```python
from build123d import *

# Parameters (mm, degrees)
F0_R     = 1.8
F0_R_2   = 1.3
F1_DEPTH = 13
F0_W     = 30
F0_H     = 12
F2_DEPTH = 3
F0_W_2   = 90
F0_H_2   = 90
F3_DEPTH = 2


with BuildPart() as f1:
    # F0 (on Top) → F1 (new body)
    with BuildSketch(Plane.XY):
        with Locations((-35, 0)):
            Circle(F0_R)
        with Locations((-35, 0)):
            Circle(F0_R_2, mode=Mode.SUBTRACT)
    extrude(amount=F1_DEPTH)



with BuildPart() as f1b:
    # F0 (on Top) → F1, piece 2 (new body)
    with BuildSketch(Plane.XY):
        with Locations((-20, 0)):
            Circle(F0_R)
        with Locations((-20, 0)):
            Circle(F0_R_2, mode=Mode.SUBTRACT)
    extrude(amount=F1_DEPTH)


with BuildPart() as f1_1:
    add(f1.part)

    add(f1b.part)  # F2 merges F1b
    # F0 (on Top) → F2 (join)
    with BuildSketch(Plane.XY):
        with Locations((-27, 0)):
            Rectangle(F0_W, F0_H)
        with Locations((-35, 0)):
            Circle(F0_R, mode=Mode.SUBTRACT)
        with Locations((-20, 0)):
            Circle(F0_R, mode=Mode.SUBTRACT)
        with Locations((-20, 0)):
            Circle(F0_R_2)
        with Locations((-35, 0)):
            Circle(F0_R_2)
    extrude(amount=F2_DEPTH)

    # F0 (on Top) → F3 (join)
    with BuildSketch(Plane.XY):
        Rectangle(F0_W_2, F0_H_2)
        with Locations((-27, 0)):
            Rectangle(F0_W, F0_H, mode=Mode.SUBTRACT)
    extrude(amount=F3_DEPTH)


solid = f1_1.part
```
For this review, take the finished solid that the model builds, in its own axes (mm). A direction names the side the tool comes from. Coordinates: 2 decimals unless noted, no trailing zeros. Loops run counter-clockwise (first coordinate to the right, second up) from the corner with the lowest first, then second, coordinate; pieces in that order, holes last.
1. Add section B-B, the plane x = -20. Give the boundary of the cut face in (y, z).
2. Insertion check: P1, Ø1.1, axis at x = -21, z = 2.5, coming from the -Y side; P2, Ø1.3, axis at x = -34.5, y = 0, coming from the +Z side; P3, Ø0.5, axis at y = -1, z = 2.5, coming from the -X side; P4, Ø6, axis at x = 0, y = -34.5, coming from the +Z side. Each pin has a flat end and moves straight along its axis. Give the tip position at first contact, or say it passes through.
3. Mouldability with a two-part tool opening along X and no side actions: class faces 3 (the flat face through (-1, 45, 1)), 4 (the flat face through (-35, 0, 3)), 5 (the flat face through (45, -1, 1)) as +X half, -X half, draft (parallel to the pull), parting line (faces both ways), or undercut.
4. Add section C-C, the plane y = 0. Give the boundary of the cut face in (x, z), then the cut area to 3 significant figures.
5. For faces 1 (the flat face through (-1, 1, 0)), 2 (the cylindrical face through (-33.283, 0.541, 7.93)), list the 3-axis set-ups (+Z, -Z, +X, -X, +Y, -Y) from which the entire face can be reached by the end or side of a thin tool; tool diameter is ignored.
6. For line 1 (Y direction, x = -35, z = 9); line 2 (Z direction, x = -41, y = -28.5); line 3 (Z direction, x = -22, y = 2), list the stretches that pass through material, from the lowest coordinate up.
7. Add section D-D, the plane x = -5.5. Give the boundary of the cut face in (y, z).
8. Add section A-A, the plane z = 10. Give the boundary of the cut face in (x, y), then the cut area to 3 significant figures.
Result:
1. outline: (-45, 0) - (45, 0) - (45, 2) - (6, 2) - (6, 3) - (1.8, 3) - (1.8, 13) - (1.3, 13) - (1.3, 3) - (-1.3, 3) - (-1.3, 13) - (-1.8, 13) - (-1.8, 3) - (-6, 3) - (-6, 2) - (-45, 2) - close
2. P1: stops at y = -45
2. P2: stops at z = 3
2. P3: stops at x = -42
2. P4: stops at z = 2
3. face 3: draft
3. face 4: undercut
3. face 5: +X half
4. outline: (-45, 0) - (45, 0) - (45, 2) - (-12, 2) - (-12, 3) - (-18.2, 3) - (-18.2, 13) - (-18.7, 13) - (-18.7, 3) - (-21.3, 3) - (-21.3, 13) - (-21.8, 13) - (-21.8, 3) - (-33.2, 3) - (-33.2, 13) - (-33.7, 13) - (-33.7, 3) - (-36.3, 3) - (-36.3, 13) - (-36.8, 13) - (-36.8, 3) - (-42, 3) - (-42, 2) - (-45, 2) - close
4. area: 230 mm2
5. face 1: -Z, +X, -X, +Y, -Y
5. face 2: +Z
6. line 1: y = -1.8 to -1.3, 1.3 to 1.8
6. line 2: z = 0 to 2
6. line 3: z = 0 to 3
7. outline: (-45, 0) - (45, 0) - (45, 2) - (-45, 2) - close
8. outline: circle Ø3.6 at (-35, 0); circle Ø3.6 at (-20, 0); hole circle Ø2.6 at (-35, 0); hole circle Ø2.6 at (-20, 0)
8. area: 9.74 mm2
